Geometry: see drawing. Coordinates: mm, zero at the bounding-box minimum. Coordinates: 2 decimals unless noted, no trailing zeros. Write each loop counter-clockwise with the first axis right and the second up, starting at its lowest first coordinate (ties: lowest second). Pieces come first, ordered by that corner, then holes. Notation, with made-up numbers: M 76.5,61.25 L 133.5,61.25 A34 ccw 133.5,96.25 Z; hole C -25,70 d8. An arc over 180 degrees is marked long. Answer as CSV lines item,"result". Start each with the question number.
1. Line query: probe 1 along X at (y, z) = (2.65, 92.5); probe 2 along X at (y, z) = (1.95, 51). Output: solid intervals per line, ascending. Write a range as [from, to].
2. Section A-A on z = 163. Return the cut outline in (x, y) (3 decimals).
3. Contact query for flat-ended pins moving along their axis: pin 1 Ø1.6 at (y, z) = (2, 33) entering from -X; pin 2 Ø1.6 at (x, y) = (270.5, 1) entering from +Z; pin 3 Ø1.6 at (y, z) = (1.5, 33.5) entering from +X. Output: stop coordinate, or through.
4. Section C-C on x = 171.5. Return the cut outline in (y, z) (3 decimals).
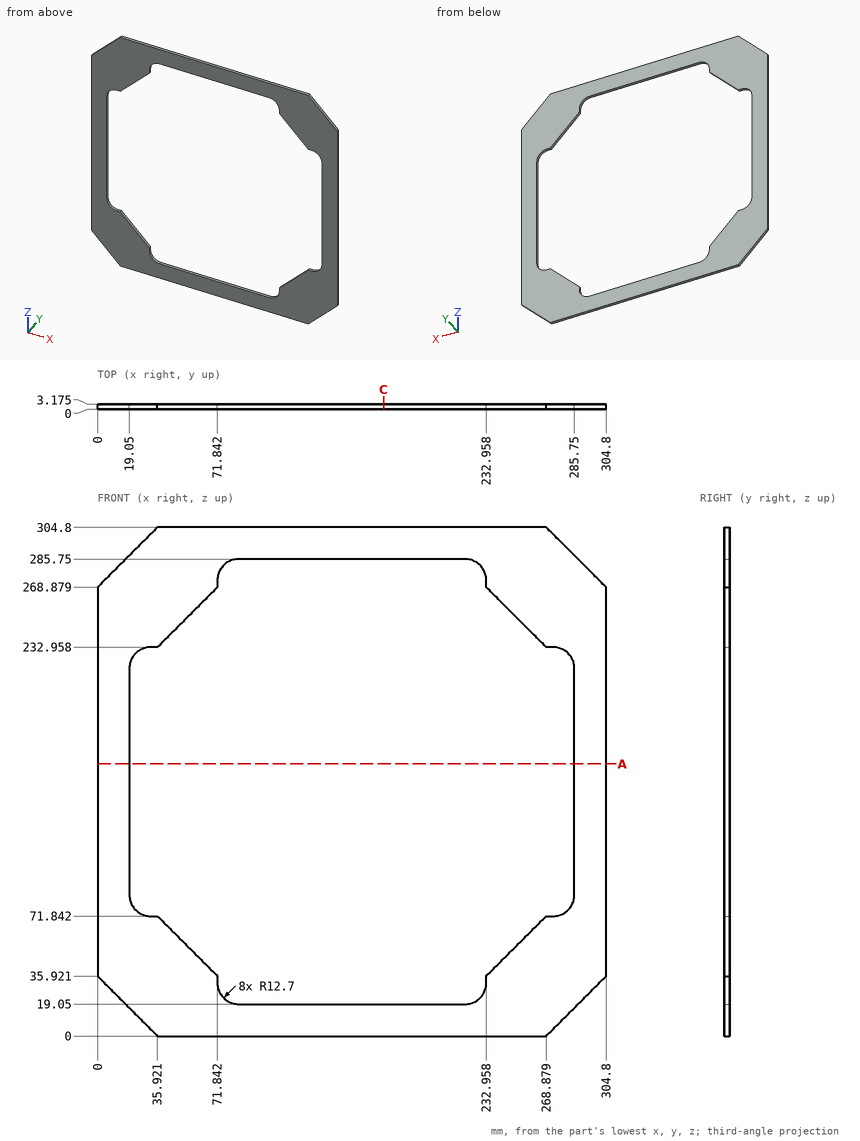
Values:
1,probe 1,"[0, 19.05], [285.75, 304.8]"
1,probe 2,"[0, 56.76], [248.04, 304.8]"
2,outline,"M 0,0 L 19.05,0 L 19.05,3.175 L 0,3.175 Z; M 285.75,0 L 304.8,0 L 304.8,3.175 L 285.75,3.175 Z"
3,pin 1,"x = 2.12"
3,pin 2,"z = 303.98"
3,pin 3,"x = 303.18"
4,outline,"M 0,0 L 3.175,0 L 3.175,19.05 L 0,19.05 Z; M 0,285.75 L 3.175,285.75 L 3.175,304.8 L 0,304.8 Z"
